Source: CAD feature listing. Evaluate the final solid. Frame: model axes, mm. Face numbers are marked on the shaded views. A direction names the side the tool comes from. Coordinates: 2 decimals unless noted, no trailing zeros. Loops run counter-clockwise (first coordinate to the right, second up) from the corner with the lowest first, then second, coordinate; pieces in that order, holes last. Notation, with made-up numbers: (-7, 73.5) - (22, 73.5) arc R9 ccw to (22, 84.5) - close; hole circle Ø5 at (70, 12). An arc over 180 degrees is marked (long way). Use one line per item in the form item = value. Start each with the question number.
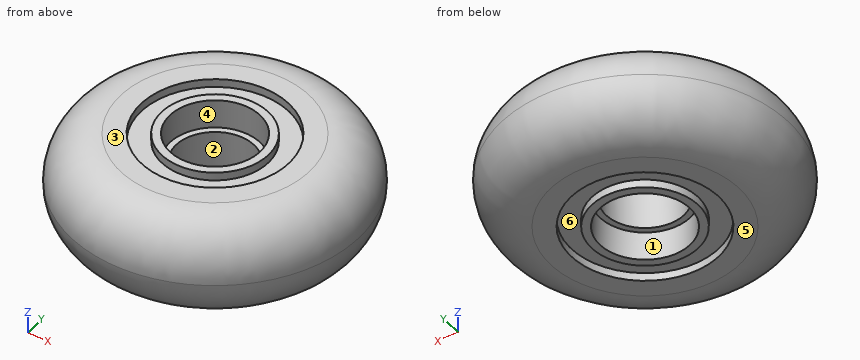
from build123d import *

# Parameters (mm, degrees)
ESQUISSE1_R             = 35
EXTRUSION1_DEPTH        = 24
CONG_1_R                = 12
CONG_2_R                = 12
ESQUISSE2_R             = 11
ENL_V_MAT_EXTRU_1_DEPTH = 7
ENL_V_START             = -7
ESQUISSE3_R             = 11
ENL_V_MAT_EXTRU_2_DEPTH = 7
ESQUISSE5_R             = 9.5
ENL_V_MAT_EXTRU_3_DEPTH = 53.335456499
ESQUISSE8_R             = 18
ESQUISSE8_R_2           = 13
ENL_V_MAT_EXTRU_4_DEPTH = 2
ENL_V_START_2           = -2
ESQUISSE9_R             = 18
ESQUISSE9_R_2           = 13
ENL_V_MAT_EXTRU_5_DEPTH = 2


with BuildPart() as part:
    # Esquisse1 → Extrusion1 (new body)
    with BuildSketch(Plane.XY):
        Circle(ESQUISSE1_R)
    extrude(amount=EXTRUSION1_DEPTH)

    # Congé1
    cong_1_edges = [part.edges().sort_by_distance(p)[0] for p in [
        (-35, 0, 24),
    ]]
    fillet(cong_1_edges, radius=CONG_1_R)

    # Congé2
    cong_2_edges = [part.edges().sort_by_distance(p)[0] for p in [
        (-35, 0, 0),
    ]]
    fillet(cong_2_edges, radius=CONG_2_R - 0.0001)  # a hair under: the kernel refuses the full size

    # Esquisse2 → Enlèv. mat.-Extru.1 (cut)
    with BuildSketch(Plane.XY.offset(24)):
        Circle(ESQUISSE2_R)
    extrude(amount=-ENL_V_MAT_EXTRU_1_DEPTH, mode=Mode.SUBTRACT)

    # Esquisse3 → Enlèv. mat.-Extru.2 (cut)
    with BuildSketch(Plane(origin=(0, 0, 0), x_dir=(-1, 0, 0), z_dir=(0, 0, -1)).offset(ENL_V_START)):
        with Locations(Location((0, 0, 0), (0, 0, 180))):
            Circle(ESQUISSE3_R)
    extrude(amount=ENL_V_MAT_EXTRU_2_DEPTH, mode=Mode.SUBTRACT)

    # Esquisse5 → Enlèv. mat.-Extru.3 (cut, through all)
    with BuildSketch(Plane.XY.offset(17)):
        Circle(ESQUISSE5_R)
    extrude(amount=-ENL_V_MAT_EXTRU_3_DEPTH, mode=Mode.SUBTRACT)

    # Esquisse8 → Enlèv. mat.-Extru.4 (cut)
    with BuildSketch(Plane(origin=(0, 0, 0), x_dir=(-1, 0, 0), z_dir=(0, 0, -1))):
        Circle(ESQUISSE8_R)
        Circle(ESQUISSE8_R_2, mode=Mode.SUBTRACT)
    extrude(amount=-ENL_V_MAT_EXTRU_4_DEPTH, mode=Mode.SUBTRACT)

    # Esquisse9 → Enlèv. mat.-Extru.5 (cut)
    with BuildSketch(Plane.XY.offset(24).offset(ENL_V_START_2)):
        with Locations(Location((0, 0, 0), (0, 0, 180))):
            Circle(ESQUISSE9_R)
        with Locations(Location((0, 0, 0), (0, 0, 180))):
            Circle(ESQUISSE9_R_2, mode=Mode.SUBTRACT)
    extrude(amount=ENL_V_MAT_EXTRU_5_DEPTH, mode=Mode.SUBTRACT)


solid = part.part
(1) Contact query for flat-ended pins moving along their axis: pin 1 (2 mm diameter, centred on y = -14, z = 20, fed in from +X); pin 2 (1 mm diameter, centred on y = -18.5, z = 21, fed in from +X); pin 3 (20 mm diameter, centred on x = 0, y = 0, fed in from +Z); pin 4 (11 mm diameter, centred on x = -3.5, y = 5, fed in from -Z). Output: stop coordinate, or through.
(2) Access query for the marked faces 4, 5 and 6. Directions: +Z, -Z, +X, -X, +Y, -Y. A direction counts if a zero-diameter tool reaches every point of the face in a straight line with its end or side. Return the directions, or none.
(3) Cut plane A-A, the plane z = 10.25. Output: boundary loops of the cut face in (x, y).
(4) Material intervals for line 1 (Y direction, x = 0, z = 1.45); line 2 (Z direction, x = 14, y = -10.5); line 3 (Y direction, x = 0, z = 5.5), sorted ascending.
(5) Mould query, pull axis Y, two halves, no side actions, for the marked faces 1, 2 and 3. Classes: +Y half, -Y half, draft (parallel to the pull), parting line (faces both ways), or undercut.
(6) Cut plane B-B, the plane z = 14.25. Output: boundary loops of the cut face in (x, y).
Recorded:
q1.pin_1 = 29.73
q1.pin_2 = 25.56
q1.pin_3 = 17
q1.pin_4 = 0
q2.face_4 = +Z
q2.face_5 = -Z, +X, -X, +Y, -Y
q2.face_6 = -Z
q3.outline = circle Ø69.74 at (0, 0); hole circle Ø19 at (0, 0)
q4.line_1 = -28.72 to -18, -13 to -11, 11 to 13, 18 to 28.72
q4.line_2 = 2 to 22
q4.line_3 = -33.09 to -11, 11 to 33.09
q5.face_1 = undercut
q5.face_2 = undercut
q5.face_3 = draft
q6.outline = circle Ø69.57 at (0, 0); hole circle Ø19 at (0, 0)
